```python
from build123d import *

# Parameters (mm, degrees)
BOSS_EXTRUDE1_DEPTH = 3
BOSS_EXTRUDE2_START = -0.5
SKETCH1_3_R         = 11
BOSS_EXTRUDE2_DEPTH = 0.5
SKETCH2_R           = 4.1
SKETCH2_R_2         = 1.1
CUT_EXTRUDE1_DEPTH  = 3.5
SKETCH2_3_R         = 2
CUT_EXTRUDE2_DEPTH  = 0.5
CIRPATTERN2_COUNT   = 4
BOSS_EXTRUDE3_START = -1.225
SKETCH1_5_R         = 11
BOSS_EXTRUDE3_DEPTH = 1.225
SKETCH3_R           = 3
SKETCH3_R_2         = 1.1
CUT_EXTRUDE3_DEPTH  = 4.225
SKETCH3_3_R         = 2
CUT_EXTRUDE4_DEPTH  = 1.225
CIRPATTERN3_COUNT   = 4


with BuildPart() as part:
    # Sketch1 → Boss-Extrude1 (new body)
    with BuildSketch(Plane.XY):
        with BuildLine():
            Line((-11, 30), (-11, -30))
            ThreePointArc((-11, -30), (0, -41), (11, -30))
            Line((11, -30), (11, 30))
            ThreePointArc((11, 30), (0, 41), (-11, 30))
        make_face()
    extrude(amount=BOSS_EXTRUDE1_DEPTH)

    # Sketch1<3> → Boss-Extrude2 (add)
    with BuildSketch(Plane.XY.offset(BOSS_EXTRUDE2_START)):
        with Locations((0, 30)):
            Circle(SKETCH1_3_R)
    extrude(amount=BOSS_EXTRUDE2_DEPTH)

    # Sketch2 → Cut-Extrude1 (cut)
    with BuildSketch(Plane.XY.offset(3)):
        with Locations((0, 30)):
            Circle(SKETCH2_R)
        with Locations((5.656854249, 35.656854249)):
            Circle(SKETCH2_R_2)
    cut_extrude1 = extrude(amount=-CUT_EXTRUDE1_DEPTH, mode=Mode.SUBTRACT)

    # Sketch2<3> → Cut-Extrude2 (cut)
    with BuildSketch(Plane.XY.offset(3)):
        with Locations((5.656854249, 35.656854249)):
            Circle(SKETCH2_3_R)
    cut_extrude2 = extrude(amount=-CUT_EXTRUDE2_DEPTH, mode=Mode.SUBTRACT)

    # CirPattern2: Cut-Extrude1, Cut-Extrude2 ×4 about axis
    cirpattern2_axis = Axis((0, 30, 0), (0, 0, 1))
    add([cut_extrude1.rotate(cirpattern2_axis, i * 360 / CIRPATTERN2_COUNT) for i in range(1, CIRPATTERN2_COUNT)], mode=Mode.SUBTRACT)
    add([cut_extrude2.rotate(cirpattern2_axis, i * 360 / CIRPATTERN2_COUNT) for i in range(1, CIRPATTERN2_COUNT)], mode=Mode.SUBTRACT)

    # Sketch1<5> → Boss-Extrude3 (add)
    with BuildSketch(Plane.XY.offset(BOSS_EXTRUDE3_START)):
        with Locations((0, -30)):
            Circle(SKETCH1_5_R)
    extrude(amount=BOSS_EXTRUDE3_DEPTH)

    # Sketch3 → Cut-Extrude3 (cut)
    with BuildSketch(Plane.XY.offset(3)):
        with Locations((0, -30)):
            Circle(SKETCH3_R)
        with Locations((5.656854249, -24.343145751)):
            Circle(SKETCH3_R_2)
    cut_extrude3 = extrude(amount=-CUT_EXTRUDE3_DEPTH, mode=Mode.SUBTRACT)

    # Sketch3<3> → Cut-Extrude4 (cut)
    with BuildSketch(Plane.XY.offset(3)):
        with Locations((5.656854249, -24.343145751)):
            Circle(SKETCH3_3_R)
    cut_extrude4 = extrude(amount=-CUT_EXTRUDE4_DEPTH, mode=Mode.SUBTRACT)

    # CirPattern3: Cut-Extrude3, Cut-Extrude4 ×4 about axis
    cirpattern3_axis = Axis((0, -30, 0), (0, 0, 1))
    add([cut_extrude3.rotate(cirpattern3_axis, i * 360 / CIRPATTERN3_COUNT) for i in range(1, CIRPATTERN3_COUNT)], mode=Mode.SUBTRACT)
    add([cut_extrude4.rotate(cirpattern3_axis, i * 360 / CIRPATTERN3_COUNT) for i in range(1, CIRPATTERN3_COUNT)], mode=Mode.SUBTRACT)


solid = part.part
```
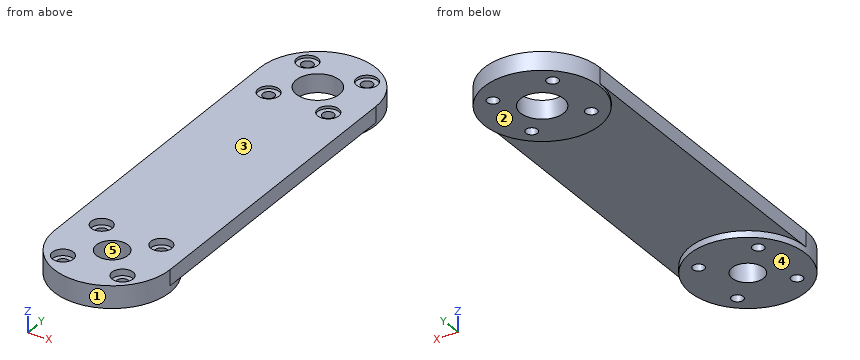
CAD build for the part. Positions are in the model's coordinates, mm. Face numbers are marked on the shaded views. A direction names the side the tool comes from. Give positions to 0.01 mm unless a question says otherwise; leave off trailing zeros. Order: outer loops, then holes, each group sorted by start corner. A loop starts at its lowest first (then second) coordinate and runs counter-clockwise, first axis right, second up. Notation, with made-up numbers: M -31,41.5 L 17,41.5 A20 ccw 17,79.5 Z; hole C 85.25,28 d10. An arc over 180 degrees is marked long. Put each result on its own line as item: value. Start each with the question number.
(1) Saw through at A-A, the plane x = 0. Write the cut outline in (y, z) (3 decimals), then the cut area to 3 significant figures.
(2) Drill centre lines: line 1 along Y through (x, z) = (-0.25, -0.15); line 2 along Y through (x, z) = (0, 2.05); line 3 along Y through (x, z) = (1, 1.7). Where is each one in solid material? Low to high.
(3) Saw through at B-B, the plane z = 0.9. Give the number of separate pieces and of enclosed holes in the cut face, then the cut area to 3 significant figures.
(4) Mould opens along Y. For the marked faces 4 and 5 say: +Y half, -Y half, draft (parallel to the pull), parting line (faces both ways), or undercut.
(5) Saw through at C-C, the plane y = -2.5. Write the cut outline in (x, z), then the cut area to 3 significant figures.
(6) Which spindle directions (+Z, -Z, +X, -X, +Y, -Y) get a long thin tool onto all of the face, cutting with end or side? Do the marked faces 1, 2 and 3. Say none if no direction does.
(7) Flat gauge pins, fed straight in: pin 1 Ø4.5 at (x, y) = (5.66, 24.34) entering from -Z; pin 2 Ø5 at (x, y) = (5.66, -35.66) entering from +Z; pin 3 Ø5 at (x, y) = (-3.5, 4.5) entering from -Z; pin 4 Ø3.5 at (x, y) = (-5.66, -35.66) entering from +Z (3 decimals). Where does each tip first touch, or does it go through?
Check result:
1. outline: M -41,-1.225 L -33,-1.225 L -33,3 L -41,3 Z; M -27,-1.225 L -19,-1.225 L -19,0 L 19,0 L 19,-0.5 L 25.9,-0.5 L 25.9,3 L -27,3 Z; M 34.1,-0.5 L 41,-0.5 L 41,3 L 34.1,3 Z
1. area: 230 mm2
2. line 1: y = -41 to -32.99, -27.01 to -19, 19 to 25.91, 34.09 to 41
2. line 2: y = -41 to -33, -27 to 25.9, 34.1 to 41
2. line 3: y = -40.95 to -32.83, -27.17 to 26.02, 33.98 to 40.95
3. separate pieces: 1
3. enclosed holes: 10
3. area: 1,590 mm2
4. face 4: draft
4. face 5: undercut
5. outline: M -11,0 L 11,0 L 11,3 L -11,3 Z
5. area: 66.0 mm2
6. face 1: -Z
6. face 2: -Z, +X, -X, +Y
6. face 3: +Z, +X, -X, +Y, -Y
7. pin 1: stops at z = -0.5
7. pin 2: stops at z = 3
7. pin 3: stops at z = 0
7. pin 4: stops at z = 1.775
